from build123d import *

# Parameters (mm, degrees)
SKETCH1_W           = 130
SKETCH1_H           = 110
BOSS_EXTRUDE1_DEPTH = 3
SKETCH2_W           = 130
SKETCH2_H           = 110
CUT_EXTRUDE1_DEPTH  = 10
SKETCH3_R           = 7
SKETCH3_R_2         = 3.451349814
SKETCH3_R_3         = 3.5
SKETCH3_R_4         = 3.533852352
CUT_EXTRUDE2_DEPTH  = 10


with BuildPart() as part:
    # Sketch1 → Boss-Extrude1 (new body)
    with BuildSketch(Plane.XY):
        Rectangle(SKETCH1_W, SKETCH1_H)
    extrude(amount=BOSS_EXTRUDE1_DEPTH)

    # Sketch2 → Cut-Extrude1 (cut)
    with BuildSketch(Plane.XY.offset(3)):
        Rectangle(SKETCH2_W, SKETCH2_H)
        with BuildLine():
            Line((-59.47576544, -53.607140846), (-63.198422227, -50.212423413))
            ThreePointArc((-63.198422227, -50.212423413), (-64.085317487, -48.731662044), (-64.00947903, -47.007282166))
            ThreePointArc((-64.00947903, -47.007282166), (-48.705948363, 1.925420221), (-12.800867901, 38.52367989))
            Line((-12.800867901, 38.52367989), (1.038853263, 44.361019449))
            ThreePointArc((1.038853263, 44.361019449), (16.438302804, 52.115303468), (31.767912546, 44.223850371))
            Line((31.767912546, 44.223850371), (45.554969528, 38.263189769))
            ThreePointArc((45.554969528, 38.263189769), (46.875270988, 37.151415741), (47.364426614, 35.496132017))
            ThreePointArc((47.364426614, 35.496132017), (60.992088303, -5.514592593), (64.85831391, -48.556955395))
            ThreePointArc((64.85831391, -48.556955395), (64.618469123, -49.190526824), (64.242583482, -49.754129754))
            Line((64.242583482, -49.754129754), (60.991812848, -53.603125765))
            ThreePointArc((60.991812848, -53.603125765), (59.545831313, -54.545662148), (57.819814936, -54.535420134))
            ThreePointArc((57.819814936, -54.535420134), (0.823909158, -49.163408252), (-56.209622322, -54.120027458))
            ThreePointArc((-56.209622322, -54.120027458), (-57.919722192, -54.354112628), (-59.47576544, -53.607140846))
        make_face(mode=Mode.SUBTRACT)
    extrude(amount=-CUT_EXTRUDE1_DEPTH, mode=Mode.SUBTRACT)

    # Sketch3 → Cut-Extrude2 (cut)
    with BuildSketch(Plane.XY.offset(3)):
        with Locations((16.353491015, 33.115492759)):
            Circle(SKETCH3_R)
        with Locations((40.35325191, 33.008362077)):
            Circle(SKETCH3_R_2)
        with Locations((-7.64626988, 33.222623441)):
            Circle(SKETCH3_R_3)
        with Locations((-40.448942317, -29.003775794)):
            Circle(SKETCH3_R)
        with Locations((-56.620414459, -46.737458118)):
            Circle(SKETCH3_R_3)
        with Locations((-24.277470176, -11.27009347)):
            Circle(SKETCH3_R_3)
        with Locations((20.598283056, -16.190449825)):
            Circle(SKETCH3_R_3)
        with Locations((38.933809649, -31.676200197)):
            Circle(SKETCH3_R)
        with Locations((57.269336242, -47.161950568)):
            Circle(SKETCH3_R_4)
    extrude(amount=-CUT_EXTRUDE2_DEPTH, mode=Mode.SUBTRACT)


solid = part.part
For this review, take the finished solid that the model builds, in its own axes (mm). Give positions to 0.01 mm unless a question says otherwise; leave off trailing zeros. Loops run counter-clockwise (first coordinate to the right, second up) from the corner with the lowest first, then second, coordinate; pieces in that order, holes last. Notation, with made-up numbers: M 56,-27 L 107,-27 A28 cw 107,7 Z; hole C 80,13 d10. An arc over 180 degrees is marked long. Put each result on its own line as item: value. Start each with the question number.
(1) Add section C-C, the plane x = -23. Write out the cut boundary in (y, z).
(2) The part is to be moulded in two halves that separate along Y. For faces 1 (the cylindrical face through (16.188, 52.115, 1.521)), 2 (the cylindrical face through (-8.102, 36.693, 1.521)), 3 (the cylindrical face through (1.626, -49.167, 1.521)), say which applies: +Y half, -Y half, draft (parallel to the pull), parting line (faces both ways), or undercut.
(3) Add section B-B, the plane x = -41. Write out the cut boundary in (y, z).
(4) Add section D-D, the plane y = 17.5. Write out the cut boundary in (x, z).
(5) Wall thickness on L1, parallel to Y at x = 21.5, z = 0.3; L2, parallel to X at y = -48, z = 2.05; L3, parallel to X at y = -30, z = 1.55: over which ranges is each line inside the solid? List them lowest first.
(6) For pin 1 (1.5 mm diameter, centred on y = -19.5, z = 1.5, fed in from +X); pin 2 (1.5 mm diameter, centred on x = 9.5, z = 2, fed in from +Y); pin 3 (1.5 mm diameter, centred on x = 29.5, z = 2, fed in from -Y), all flat-tipped, find the tip position at first contact; note any pin that passes through.
(7) Add section A-A, the plane z = 1.65. Give the number of separate pieces and of enclosed holes in the cut face, then the cut area to 3 significant figures.
Result:
1. outline: M -49.97,0 L -14.53,0 L -14.53,3 L -49.97,3 Z; M -8.01,0 L 31.31,0 L 31.31,3 L -8.01,3 Z
2. face 1: +Y half
2. face 2: undercut
2. face 3: -Y half
3. outline: M -51.78,0 L -35.98,0 L -35.98,3 L -51.78,3 Z; M -22.03,0 L 13.15,0 L 13.15,3 L -22.03,3 Z
4. outline: M -37.41,0 L 54.65,0 L 54.65,3 L -37.41,3 Z
5. L1: y = -49.91 to -19.57, -12.81 to 28.37, 37.86 to 51.41
5. L2: x = -64.18 to -59.88, -53.36 to 53.84, 60.7 to 64.87
5. L3: x = -61.52 to -47.38, -33.52 to 32.14, 45.73 to 64.42
6. pin 1: stops at x = 63.45
6. pin 2: stops at y = 51.11
6. pin 3: stops at y = -50.64
7. separate pieces: 1
7. enclosed holes: 9
7. area: 9,390 mm^2
